from build123d import *

# Parameters (mm, degrees)
SKETCH1_R           = 2.5
SKETCH1_R_2         = 6
SKETCH1_R_3         = 2
BOSS_EXTRUDE1_DEPTH = 5
FILLET1_R           = 5


with BuildPart() as part:
    # Sketch1 → Boss-Extrude1 (new body)
    with BuildSketch(Plane.XY):
        Polygon((0, 0), (180, 0), (180, -19), (50, -19), (50, -90), (0, -90), align=None)
        with Locations((135, -9.5)):
            Circle(SKETCH1_R, mode=Mode.SUBTRACT)
        with Locations((165, -9.5)):
            Circle(SKETCH1_R, mode=Mode.SUBTRACT)
        with Locations((25, -68.5)):
            Circle(SKETCH1_R_2, mode=Mode.SUBTRACT)
        with Locations((7.5, -68.5)):
            Circle(SKETCH1_R_3, mode=Mode.SUBTRACT)
        with Locations((42.5, -68.5)):
            Circle(SKETCH1_R_3, mode=Mode.SUBTRACT)
    extrude(amount=BOSS_EXTRUDE1_DEPTH)

    # Fillet1
    fillet1_edges = [part.edges().sort_by_distance(p)[0] for p in [
        (0, 0, 2.5),
        (180, 0, 2.5),
        (180, -19, 2.5),
        (50, -19, 2.5),
        (50, -90, 2.5),
        (0, -90, 2.5),
    ]]
    fillet(fillet1_edges, radius=FILLET1_R)


solid = part.part
Geometry: final body of the model. Coordinates: model frame, mm. A direction names the side the tool comes from. Coordinates: 2 decimals unless noted, no trailing zeros. Order: outer loops, then holes, each group sorted by start corner. A loop starts at its lowest first (then second) coordinate and runs counter-clockwise, first axis right, second up.
(1) First-contact query: pin 1 (1.5 mm diameter, centred on x = 74.5, z = 3, fed in from -Y); pin 2 (1.5 mm diameter, centred on y = -28, z = 1, fed in from +X). Flat tips, straight axial feed; report the tip coordinate or a pass-through.
(2) Section query B-B (z = 3.5). Return the cut outline in (x, y).
(3) Material intervals for probe 1 along Y at (x, z) = (42.5, 2.3); probe 2 along Y at (x, z) = (135, 1.15); probe 3 along X at (y, z) = (-82, 2.65), sorted ascending.
(4) Access query for faces 1 (the face through (50, -54, 2)), 2 (the face through (0, -46, 2)). Directions: +Z, -Z, +X, -X, +Y, -Y. A direction counts if a zero-diameter tool reaches every point of the face in a straight line with its end or side. Return the directions, or none.
(5) Section query C-C (y = -9.5). Return the cut outline in (x, z).
(6) Draft query along X for faces 3 (the face through (51, -14, 5)), 4 (the face through (2, -1, 3)), 5 (the face through (48, -89, 3)), 6 (the face through (7.24, -66.517, 2.465)). Return one class per face: pulls with the +X half, pulls with the -X half, needs draft (parallel to the pull), parting line crosses it, or undercut.
(7) Section query D-D (x = 165). Return the cut outline in (y, z).
(8) Section query A-A (x = 42.5). Return the cut outline in (y, z).
Solution:
1. pin 1: stops at y = -19
1. pin 2: stops at x = 50
2. outline: (0, -85) arc R5 ccw to (5, -90) - (45, -90) arc R5 ccw to (50, -85) - (50, -24) arc R5 cw to (55, -19) - (175, -19) arc R5 ccw to (180, -14) - (180, -5) arc R5 ccw to (175, 0) - (5, 0) arc R5 ccw to (0, -5) - close; hole circle Ø4 at (7.5, -68.5); hole circle Ø12 at (25, -68.5); hole circle Ø4 at (42.5, -68.5); hole circle Ø5 at (135, -9.5); hole circle Ø5 at (165, -9.5)
3. probe 1: y = -90 to -70.5, -66.5 to 0
3. probe 2: y = -19 to -12, -7 to 0
3. probe 3: x = 0 to 50
4. face 1: +Z, -Z, +X, -Y
4. face 2: +Z, -Z, -X, +Y, -Y
5. outline: (0, 0) - (132.5, 0) - (132.5, 5) - (0, 5) - close; (137.5, 0) - (162.5, 0) - (162.5, 5) - (137.5, 5) - close; (167.5, 0) - (180, 0) - (180, 5) - (167.5, 5) - close
6. face 3: needs draft
6. face 4: pulls with the -X half
6. face 5: pulls with the +X half
6. face 6: undercut
7. outline: (-19, 0) - (-12, 0) - (-12, 5) - (-19, 5) - close; (-7, 0) - (0, 0) - (0, 5) - (-7, 5) - close
8. outline: (-90, 0) - (-70.5, 0) - (-70.5, 5) - (-90, 5) - close; (-66.5, 0) - (0, 0) - (0, 5) - (-66.5, 5) - close
